Input: part model. Units: mm. Frame: model coordinates. Face numbers are marked on the shaded views. A direction names the side the tool comes from. Round coordinates to 2 decimals unless told otherwise and drop trailing zeros. Write each loop counter-clockwise with the first axis right and the second up, starting at its lowest first coordinate (ties: lowest second). Pieces come first, ordered by that corner, then holes. Notation, with made-up numbers: (40.5, 31) -> (60.5, 31) arc R17 ccw to (60.5, 51) -> close; hole circle Ø9 at (-32, 15). An arc over 180 degrees is marked (long way). Use CSV: the item, a comma, the result in double quotes.
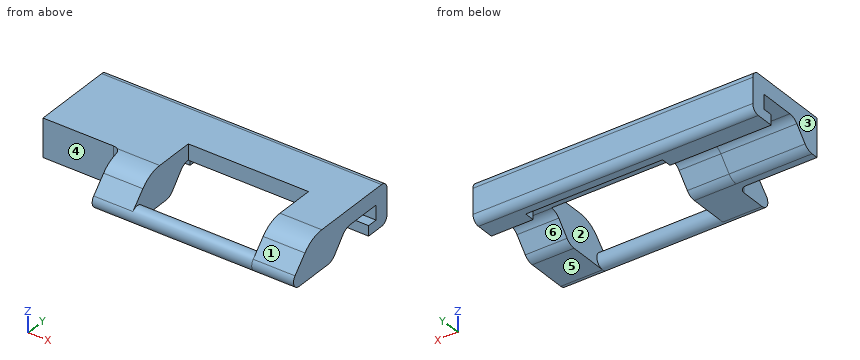
```python
from build123d import *

# Parameters (mm, degrees)
F0_R      = 1.5875
F1_DEPTH  = 12.065
F3_DEPTH  = 8.382
F6_DEPTH  = 24.13
F7_R      = 2.54
F9_DEPTH  = 15.24
F11_DEPTH = 0.508
F12_R     = 1.524
F13_W     = 2.032
F13_H     = 2.032
F14_DEPTH = 3.302
F15_R     = 1.5875


with BuildPart() as f1:
    # F0 (on Right) → F1 (new body)
    with BuildSketch(Plane.YZ):
        Circle(F0_R)
    extrude(amount=F1_DEPTH)

    # F2 (on face) → F3 (join)
    with BuildSketch(Plane.YZ.offset(12.065)):
        with BuildLine():
            Line((24.3205, -2.032), (24.3205, 6.096))
            Line((24.3205, 6.096), (6.2485151547, 6.096))
            ThreePointArc((6.2485151547, 6.096), (3.7025695222, 5.5632726287), (1.5838033934, 4.0544758539))
            Line((1.5838033934, 4.0544758539), (-1.1661779403, 1.0771189635))
            ThreePointArc((-1.1661779403, 1.0771189635), (-1.4543181572, -0.6364864081), (0, -1.5875))
            Line((0, -1.5875), (9.0805, -1.5875))
            Line((9.0805, -1.5875), (12.8905, 2.921))
            Line((12.8905, 2.921), (21.2725, 2.921))
            Line((21.2725, 2.921), (21.2725, 0))
            Line((21.2725, 0), (19.2405, 0))
            Line((19.2405, 0), (19.2405, -2.032))
            Line((19.2405, -2.032), (24.3205, -2.032))
        make_face()
    extrude(amount=F3_DEPTH)

    # F4: F1 across plane


with BuildPart() as f1_1:
    add(f1.part)
    add(f1.part.mirror(Plane.YZ))

    # F5 (on face) → F6 (join, through all)
    with BuildSketch(Plane.YZ.offset(-12.065)):
        Polygon((24.3205, -2.032), (24.3205, 6.096), (14.1605, 6.096), (14.1605, 2.921), (21.2725, 2.921), (21.2725, -2.032), align=None)
    extrude(amount=F6_DEPTH)

    # F7
    f7_edges = [f1_1.edges().sort_by_distance(p)[0] for p in [
        (16.256, 9.0805, -1.5875),
        (16.256, 12.8905, 2.921),
        (-16.256, 9.0805, -1.5875),
        (-16.256, 12.8905, 2.921),
    ]]
    fillet(f7_edges, radius=F7_R)

    # F8 (on face) → F9 (join)
    with BuildSketch(Plane(origin=(-20.447, 0, 0), x_dir=(0, -1, 0), z_dir=(-1, 0, 0))):
        with BuildLine():
            Line((-6.5405, 6.096), (-24.3205, 6.096))
            Line((-24.3205, 6.096), (-24.3205, -2.032))
            Line((-24.3205, -2.032), (-19.2405, -2.032))
            Line((-19.2405, -2.032), (-19.2405, 0))
            Line((-19.2405, 0), (-21.2725, 0))
            Line((-21.2725, 0), (-21.2725, 2.921))
            Line((-21.2725, 2.921), (-14.0695243298, 2.921))
            ThreePointArc((-14.0695243298, 2.921), (-13.0000966588, 2.6848933258), (-12.1294871065, 2.020468076))
            Line((-12.1294871065, 2.020468076), (-9.8415128935, -0.686968076))
            ThreePointArc((-9.8415128935, -0.686968076), (-8.9709033412, -1.3513933258), (-7.9014756702, -1.5875))
            Line((-7.9014756702, -1.5875), (-6.5405, -1.5875))
            Line((-6.5405, -1.5875), (-6.5405, 6.096))
        make_face()
    extrude(amount=F9_DEPTH)

    # F10 (on face) → F11 (cut)
    with BuildSketch(Plane(origin=(-20.447, 0, 0), x_dir=(0, -1, 0), z_dir=(-1, 0, 0))):
        with BuildLine():
            ThreePointArc((-1.5838033934, 4.0544758539), (-3.7025695222, 5.5632726287), (-6.2485151547, 6.096))
            Line((-6.2485151547, 6.096), (-6.5405, 6.096))
            Line((-6.5405, 6.096), (-6.5405, -1.5875))
            Line((-6.5405, -1.5875), (0, -1.5875))
            ThreePointArc((0, -1.5875), (1.4543181572, -0.6364864081), (1.1661779403, 1.0771189635))
            Line((1.1661779403, 1.0771189635), (-1.5838033934, 4.0544758539))
        make_face()
    extrude(amount=-F11_DEPTH, mode=Mode.SUBTRACT)

    # F12
    f12_edges = [f1_1.edges().sort_by_distance(p)[0] for p in [
        (-7.62, 24.3205, 6.096),
        (-7.62, 24.3205, -2.032),
    ]]
    fillet(f12_edges, radius=F12_R)

    # F13 (on face) → F14 (cut)
    with BuildSketch(Plane.YZ.offset(-12.065)):
        with Locations((20.2565, -1.016)):
            Rectangle(F13_W, F13_H)
    extrude(amount=-F14_DEPTH, mode=Mode.SUBTRACT)

    # F15
    f15_edges = [f1_1.edges().sort_by_distance(p)[0] for p in [
        (-19.939, 6.5405, 2.25425),
    ]]
    fillet(f15_edges, radius=F15_R)


solid = f1_1.part
```
Item 1: Set-up query: the marked faces 4, 5 and 6. Return all of +Z, -Z, +X, -X, +Y, -Y with unobstructed straight access to the full face (end or side cutting, diameter ignored); none if empty.
Worked answers:
face 4,"+Z, -Z, -X, -Y"
face 5,"-Z, +X, -X, -Y"
face 6,"-Z, +X, -X"
Item 2: Pull-direction query (X, two-part tool) for the marked faces 1, 2 and 3; classes: +X half, -X half, draft (parallel to the pull), parting line (faces both ways), or undercut.
Worked answers:
face 1,"draft"
face 2,"undercut"
face 3,"-X half"
Item 3: Section query A-A on x = 8.5. Return the cut outline in (y, z) (1 decimal), plus the area to 3 significant figures.
Worked answers:
outline,"circle Ø3.2 at (0, 0); (14.2, 2.9) -> (21.3, 2.9) -> (21.3, -2) -> (22.8, -2) arc R1.5 ccw to (24.3, -0.5) -> (24.3, 4.6) arc R1.5 ccw to (22.8, 6.1) -> (14.2, 6.1) -> close"
area,"54.3 mm²"
Item 4: Section query C-C on z = 0.5. Return the cut outline in (x, y) (1 decimal).
Worked answers:
outline,"(-35.7, 6.5) -> (-21.5, 6.5) arc R1.6 cw to (-19.9, 5) -> (-19.9, -1.5) -> (20.4, -1.5) -> (20.4, 10.8) -> (12.1, 10.8) -> (12.1, 1.5) -> (-12.1, 1.5) -> (-12.1, 10.8) -> (-35.7, 10.8) -> close; (-35.7, 21.3) -> (20.4, 21.3) -> (20.4, 24.3) -> (-35.7, 24.3) -> close"
Item 5: Line query: line 1 (X direction, y = 9, z = 2.5) (3 decimals); line 2 (X direction, y = 5, z = -0.75) (3 decimals); line 3 (Y direction, x = 5, z = 4.25). Output: solid intervals per line, ascending.
Worked answers:
line 1,"x = -35.687 to -12.065, 12.065 to 20.447"
line 2,"x = -19.94 to -12.065, 12.065 to 20.447"
line 3,"y = 14.16 to 24.32"
Item 6: First-contact query: pin 1 Ø3.5 at (x, y) = (-8.5, 17.5) entering from -Z; pin 2 Ø2 at (y, z) = (0.5, 1.5) entering from -X; pin 3 Ø2.5 at (x, y) = (-20.5, 4) entering from -Z. Flat tips, straight axial feed; report the tip coordinate or a pass-through.
Worked answers:
pin 1,"stops at z = 2.92"
pin 2,"stops at x = -19.94"
pin 3,"stops at z = -1.59"
Item 7: Section query B-B on y = 7.25. Return the cut outline in (x, z) (1 decimal).
Worked answers:
outline,"(-35.7, -1.6) -> (-12.1, -1.6) -> (-12.1, 6.1) -> (-35.7, 6.1) -> close; (12.1, -1.6) -> (20.4, -1.6) -> (20.4, 6.1) -> (12.1, 6.1) -> close"
